```python
from build123d import *

# Parameters (mm, degrees)
F2_R    = 5.08
F3_SIZE = 1


with BuildPart() as f1:
    # F0 (on Front) → F1 (revolve)
    with BuildSketch(Plane.XZ):
        Polygon((7.780209, 58.772128), (0, 58.772128), (0, 0), (19.34539, 0), (19.34539, 37.954811), (7.780209, 47.627505), align=None)
    revolve(axis=Axis((0, 0, 29.386064), (0, 0, 1)))

    # F2
    f2_edges = [f1.edges().sort_by_distance(p)[0] for p in [
        (-7.780209, 0, 58.772128),
    ]]
    fillet(f2_edges, radius=F2_R)

    # F3
    f3_edges = [f1.edges().sort_by_distance(p)[0] for p in [
        (-19.34539, 0, 0),
    ]]
    chamfer(f3_edges, length=F3_SIZE)


solid = f1.part
```
For this review, take the finished solid that the model builds, in its own axes (mm). A direction names the side the tool comes from. Coordinates: 2 decimals unless noted, no trailing zeros. Loops run counter-clockwise (first coordinate to the right, second up) from the corner with the lowest first, then second, coordinate; pieces in that order, holes last.
1. Insertion check: P1, Ø4, axis at x = -7.5, y = -2.5, coming from the +Z side; P2, Ø8, axis at x = -12, y = 14.5, coming from the -Z side; P3, Ø1, axis at x = -11, y = 9, coming from the +Z side; P4, Ø4, axis at x = 0, z = 42, coming from the -Y side. Each pin has a flat end and moves straight along its axis. Give the tip position at first contact, or say it passes through.
2. Add section B-B, the plane z = 43.5. Give the boundary of the cut face in (x, y), then the cut area to 3 significant figures.
3. For faces 1 (the cylindrical face through (-1.013, 7.714, 50.702)), 2 (the flat face through (0, 0, 0)), list the 3-axis set-ups (+Z, -Z, +X, -X, +Y, -Y) from which the entire face can be reached by the end or side of a thin tool; tool diameter is ignored.
4. For line 1 (Y direction, x = -17, z = 35); line 2 (X direction, y = 13, z = 17.5); line 3 (Z direction, x = 3.5, y = 13), list the stretches that pass through material, from the lowest coordinate up.
5. Add section A-A, the plane z = 20. Give the boundary of the cut face in (x, y).
Result:
1. P1: stops at z = 57.63
1. P2: stops at z = 0
1. P3: stops at z = 42.67
1. P4: stops at y = -16.9
2. outline: circle Ø25.43 at (0, 0)
2. area: 508 mm2
3. face 1: +Z
3. face 2: -Z, +X, -X, +Y, -Y
4. line 1: y = -9.23 to 9.23
4. line 2: x = -14.33 to 14.33
4. line 3: z = 0 to 42.87
5. outline: circle Ø38.69 at (0, 0)
